Source: CAD feature listing. Evaluate the final solid. Frame: model axes, mm. Face numbers are marked on the shaded views. A direction names the side the tool comes from. Round coordinates to 2 decimals unless told otherwise and drop trailing zeros. Write each loop counter-clockwise with the first axis right and the second up, starting at its lowest first coordinate (ties: lowest second). Pieces come first, ordered by that corner, then holes.
Autodesk Inventor part; units mm, degrees
ref_plane "YZ Plane" through (0, 0, 0) normal (1, 0, 0) x (0, 1, 0)
ref_plane "XZ Plane" through (0, 0, 0) normal (0, 1, 0) x (-1, 0, 0)
ref_plane "XY Plane" through (0, 0, 0) normal (0, 0, 1) x (1, 0, 0)
sketch "Sketch1" plane through (0, 0, 0) normal (0, 1, 0) x (-1, 0, 0)
  line L0 (0, 0) -> (-48.5, 0)
  line L1 (-48.5, 0) -> (-48.5, -55)
  line L2 (-48.5, -55) -> (0, -55)
  line L3 (0, -55) -> (0, 0)
  line L4 (1.5, 1.5) -> (-50, 1.5)
  line L5 (-50, 1.5) -> (-50, -56.5)
  line L6 (-50, -56.5) -> (1.5, -56.5)
  line L7 (1.5, -56.5) -> (1.5, 1.5)
  dimension "d0" = 55
  dimension "d1" = 48.5
  dimension "d2" = 51.5
  dimension "d3" = 58
  dimension "d4" = 1.5
  dimension "d5" = 1.5
extrude "Extrusion1" add sketch "Sketch1" against normal blind 1.5 contours L3 L2 L1 L0 | L7 L6 L5 L4
sketch "Sketch2" plane through (0, 0, 0) normal (0, 1, 0) x (1, 0, 0)
  line L0 (-1.5, -1.5) -> (50, -1.5)
  line L1 (50, 56.5) -> (-1.5, 56.5)
  line L2 (-1.5, 56.5) -> (-1.5, -1.5)
  line L3 (0, 0) -> (50, 0)
  line L4 (50, 55) -> (0, 55)
  line L5 (0, 55) -> (0, 0)
  line L6 (50, 0) -> (50, -1.5)
  line L7 (50, 56.5) -> (50, -1.5)
  line L8 (50, 55) -> (50, 56.5)
  line L9 (-1.5, 56.5) -> (50, 56.5)
  dimension "d8" = 55
extrude "Extrusion2" add sketch "Sketch2" along normal blind 28 contours L2 L1 L7 L4 L5 L3 L6 L0
sketch "Sketch3" plane through (0, 28, 0) normal (0, 1, 0) x (1, 0, 0)
  line L0 (-1.5, 56.5) -> (50, 56.5)
  line L1 (50, 56.5) -> (50, -1.5)
  line L2 (50, -1.5) -> (-1.5, -1.5)
  line L3 (-1.5, -1.5) -> (-1.5, 56.5)
  point P0 (0, 0)
extrude "Extrusion3" add sketch "Sketch3" along normal blind 1.5
fillet "Fillet1" radius 1 8 edges at (24.25, 29.5, 1.5) (24.25, 29.5, -56.5) (-1.5, 29.5, -27.5) (-1.5, 14, 1.5) (24.25, -1.5, 1.5) (-1.5, -1.5, -27.5) (24.25, -1.5, -56.5) (-1.5, 14, -56.5)
sketch "Sketch4" plane through (0, 0, 0) normal (1, 0, 0) x (0, 0, -1)
  line L0 (15, 0) -> (25, 0)
  line L1 (25, 0) -> (25, 3.3)
  line L2 (25, 3.3) -> (15, 3.3)
  line L3 (15, 3.3) -> (15, 0)
  line L4 (0, 0) -> (0, 28)
  dimension "d14" = 3.3
  dimension "d15" = 10
  dimension "d16" = 15
extrude "Extrusion4" add sketch "Sketch4" along normal blind 10
ref_plane "Work Plane1" through (50, 0, -27.5) normal (0, 0, -1) x (-1, 0, 0)
sketch "Sketch5" plane through (50, 0, 0) normal (0, 0, -1) x (-1, 0, 0)
  line L0 (10, 5.5) -> (35, 5.5)
  line L1 (35, 5.5) -> (35, 4.5)
  line L2 (35, 4.5) -> (10, 4.5)
  line L3 (10, 4.5) -> (10, 5.5)
  line L4 (50, 0) -> (0, 0)
  line L5 (50, 0) -> (50, 28)
  line L6 (0, 0) -> (0, 28)
  dimension "d20" = 1
  dimension "d21" = 4.5
  dimension "d22" = 15
  dimension "d23" = 10
extrude "Extrusion5" add sketch "Sketch5" along normal blind 2
mirror "Mirror1" about plane through (50, 0, -27.5) normal (0, 0, -1) of "Extrusion5"
sketch "Sketch6" plane through (0, 0, -55) normal (1, 0, 0) x (0, 0, -1)
  line L0 (-22, 1) -> (-10, 1)
  line L1 (-10, 1) -> (-10, 14)
  line L2 (-10, 14) -> (-22, 14)
  line L3 (-22, 14) -> (-22, 1)
  line L4 (0, 0) -> (-30, 0)
  line L5 (0, 0) -> (0, 28)
  point P0 (-55, 0)
  dimension "d26" = 1
  dimension "d27" = 22
  dimension "d28" = 10
  dimension "d29" = 13
extrude "Extrusion6" cut sketch "Sketch6" against normal blind 2
fillet "Fillet2" radius 0.5 4 edges at (-0.75, 1, -33) (-0.75, 14, -33) (-0.75, 14, -45) (-0.75, 1, -45)
sketch "Sketch7" plane through (50, -0.5, 1.5) normal (1, 0, 0) x (0, 0, -1)
  line L0 (0, 0) -> (0, 29)
  line L1 (0, 16.5) -> (58, 16.5)
  line L2 (58, 16.5) -> (58, 30)
  line L3 (58, 30) -> (0, 30)
  line L4 (0, 30) -> (0, 16.5)
  line L5 (0.75, 29.25) -> (57.25, 29.25)
  line L6 (57.25, 29.25) -> (57.25, 16.5)
  line L7 (57.25, 16.5) -> (0.75, 16.5)
  line L8 (0.75, 16.5) -> (0.75, 29.25)
  line L9 (58, 0) -> (58, 29)
  line L10 (56.5, 0.5) -> (56.5, 28.5)
  line L11 (1.5, 28.5) -> (56.5, 28.5)
  line L12 (56.5, 28.5) -> (56.5, 16.5)
  line L13 (56.5, 16.5) -> (1.5, 16.5)
  line L14 (1.5, 16.5) -> (1.5, 28.5)
  line L15 (1, 30) -> (57, 30)
  point P0 (1.5, 0.5)
  dimension "d33" = 0.75
  dimension "d34" = 0.75
  dimension "d35" = 0
  dimension "d36" = 0.75
  dimension "d37" = 0
  dimension "d38" = 0.75
  dimension "d39" = 0.75
  dimension "d40" = 12.75
  dimension "d41" = 0
extrude "Extrusion7" cut sketch "Sketch7" against normal blind 3 contours L0 L4 L3 L2 L1 L6 L5 L8
fillet "Fillet3" radius 1 2 edges at (48.5, 28.75, -55.75) (48.5, 28.75, 0.75)
sketch "Sketch8" plane through (50, -1.5, 0.5) normal (1, 0, 0) x (0, 0, -1)
  line L0 (57.0002, 13.25) -> (-0.9998, 13.25)
  line L1 (-0.9998, 13.25) -> (-0.9998, 0.75)
  line L2 (-0.9998, 0.75) -> (57.0002, 0.75)
  line L3 (57.0002, 0.75) -> (57.0002, 13.25)
  line L4 (56, 0) -> (0, 0)
  line L5 (-0.2498, 13.25) -> (56.2502, 13.25)
  line L6 (56.2502, 13.25) -> (56.2502, 0.75)
  line L7 (56.2502, 0.75) -> (-0.2498, 0.75)
  line L8 (-0.2498, 0.75) -> (-0.2498, 13.25)
  line L9 (0.5, 13.25) -> (55.5, 13.25)
  line L10 (55.5, 13.25) -> (55.5, 1.5)
  line L11 (55.5, 1.5) -> (0.5, 1.5)
  line L12 (0.5, 1.5) -> (0.5, 13.25)
  dimension "d45" = 58
  dimension "d46" = 12.5
  dimension "d47" = 0.75
  dimension "d48" = 0
  dimension "d49" = 0.75
  dimension "d50" = 0.75
extrude "Extrusion8" cut sketch "Sketch8" against normal blind 3 contours L6 L2 L8 L0 L12 L11 L10
sketch "Sketch9" plane through (50, -0.5, -56.5) normal (0, 0, -1) x (-1, 0, 0)
  line L0 (3, 12.25) -> (5, 12.25)
  line L1 (5, 12.25) -> (5, 25)
  line L2 (5, 25) -> (3, 25)
  line L3 (3, 25) -> (3, 12.25)
  line L4 (5, 12.25) -> (0, 12.25)
  line L5 (0, 12.25) -> (0, 5)
  line L6 (0, 5) -> (5, 5)
  line L7 (5, 5) -> (5, 12.25)
  line L8 (0, 0) -> (0, 16.5)
  point P0 (50, 0.5)
  point P1 (3, 30)
  point P2 (0, -1)
  dimension "d60" = 2
  dimension "d61" = 12.75
  dimension "d62" = 5
  dimension "d63" = 5
  dimension "d64" = 7.25
  dimension "d65" = 0
extrude "Extrusion9" add sketch "Sketch9" along normal blind 5
fillet "Fillet4" radius 1 2 edges at (46, 24.5, -61.5) (47.5, 4.5, -61.5)
sketch "Sketch10" plane through (47, -0.5, 1.5) normal (1, 0, 0) x (0, 0, -1)
  circle A0 centre (60.5, 21.5) radius 1.5
  line L0 (63, 24) -> (63, 12.25)
  line L1 (58, 25) -> (62, 25)
  point P0 (1.5, 0.5)
  dimension "d69" = 3
  dimension "d70" = 2.5
  dimension "d71" = 3.5
extrude "Extrusion10" cut sketch "Sketch10" against normal blind 2
sketch "Sketch11" plane through (50, -1.5, 0.5) normal (1, 0, 0) x (0, 0, -1)
  circle A0 centre (59.5, 9.5) radius 1.5
  line L0 (57, 6) -> (61, 6)
  line L1 (62, 13.25) -> (62, 7)
  point P0 (0.5, 1.5)
  dimension "d74" = 3
  dimension "d75" = 3.5
  dimension "d76" = 2.5
extrude "Extrusion11" cut sketch "Sketch11" against normal blind 5
mirror "Mirror2" about plane through (50, 0, -27.5) normal (0, 0, -1) of "Extrusion9", "Extrusion11", "Fillet4", "Extrusion10"
equation "\"d34\" = d33"
equation "\"d36\" = d33"
equation "\"d38\" = d36"
equation "\"d39\" = d33"
properties part number "sensor2t"
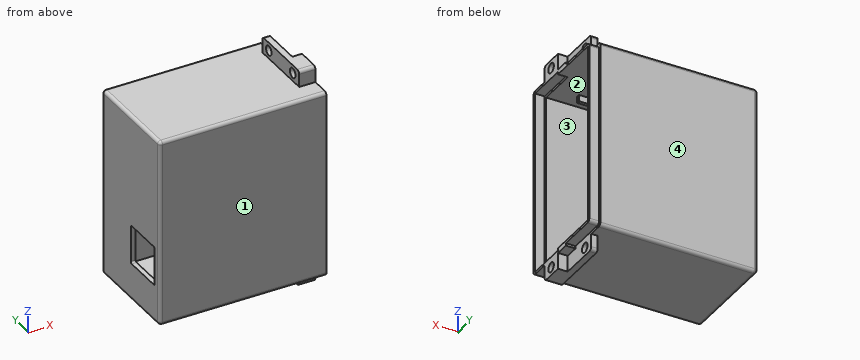
Q1. Mould query, pull axis Z, two halves, no side actions, for the marked faces 1 and 2. Classes: pulls with the +Z half, pulls with the -Z half, needs draft (parallel to the pull), parting line crosses it, or undercut.
Q2. Line query: line 1 (Y direction, x = 46, z = -59); line 2 (Y direction, x = 49, z = 4); line 3 (Y direction, x = 5.5, z = -4.5). Output: solid intervals per line, ascending.
Q3. Section query A-A, the plane z = -59. Output: boundary loops of the cut face in (x, y).
Q4. Section query B-B, the plane y = 21. Output: boundary loops of the cut face in (x, z), and give its area (3 significant figures).
Q5. Set-up query: the marked faces 3 and 4. Return all of +Z, -Z, +X, -X, +Y, -Y with unobstructed straight access to the full face (end or side cutting, diameter ignored); none if empty.
Q6. Pin query (flat end, axial travel): P1, Ø1.5, axis at y = 18.5, z = -8.5, coming from the +X side; P2, Ø1.6, axis at x = -0.5, y = 9.5, coming from the +Z side; P3, Ø2.5, axis at y = 8, z = -59, coming from the -X side; P4, Ø1, axis at y = 2.5, z = -18.5, coming from the +X side. Return the tip coordinate at first contact, or that it passes through.
Q7. Section query D-D, the plane x = 17.5. Output: boundary loops of the cut face in (y, z).
Q8. Section query C-C, the plane y = 8. Give the number of separate pieces and of enclosed holes in the cut face, and give its area (3 significant figures).
Filled in:
1. face 1: needs draft
1. face 2: undercut
2. line 1: y = 4.5 to 6.5, 9.5 to 19.5, 22.5 to 24.5
2. line 2: y = 4.5 to 6.5, 9.5 to 11.75
2. line 3: y = -1.5 to 0, 28 to 29.5
3. outline: (45, 4.5) - (50, 4.5) - (50, 6.5) - (45, 6.5) - close; (45, 9.5) - (50, 9.5) - (50, 11.75) - (47, 11.75) - (47, 19.5) - (45, 19.5) - close; (45, 22.5) - (47, 22.5) - (47, 24.5) - (45, 24.5) - close
4. outline: (-1.5, -55.5) arc R1 ccw to (-0.5, -56.5) - (45, -56.5) - (45, -57.5) - (47, -57.5) - (47, -55.75) - (50, -55.75) - (50, -55) - (0, -55) - (0, 0) - (50, 0) - (50, 0.75) - (47, 0.75) - (47, 2.5) - (45, 2.5) - (45, 1.5) - (-0.5, 1.5) arc R1 ccw to (-1.5, 0.5) - close; (45, -61.5) - (47, -61.5) - (47, -60.5) - (45, -60.5) - close; (45, 5.5) - (47, 5.5) - (47, 6.5) - (45, 6.5) - close
4. area: 240 mm2
5. face 3: +X
5. face 4: +Z, -Z, +X, -X, +Y
6. P1: stops at x = 0
6. P2: stops at z = 1.5
6. P3: passes through
6. P4: stops at x = 10
7. outline: (-1.5, -55.5) arc R1 ccw to (-0.5, -56.5) - (28.5, -56.5) arc R1 ccw to (29.5, -55.5) - (29.5, 0.5) arc R1 ccw to (28.5, 1.5) - (-0.5, 1.5) arc R1 ccw to (-1.5, 0.5) - close; hole (0, -55) - (4.5, -55) - (4.5, -53) - (5.5, -53) - (5.5, -55) - (28, -55) - (28, 0) - (5.5, 0) - (5.5, -2) - (4.5, -2) - (4.5, 0) - (0, 0) - close
8. separate pieces: 4
8. enclosed holes: 0
8. area: 234 mm2
